Answer from the drawing. Dimensions are ordinates in mm from the lowest x, y and z of the part. Round coordinates to 2 decimals unless told otherwise and drop trailing zeros. Order: outer loops, then holes, each group sorted by start corner. A loop starts at its lowest first (then second) coordinate and runs counter-clockwise, first axis right, second up. Notation, with made-up numbers: (36.25, 36) - (61.25, 36) arc R25 cw to (61.25, 61) - close; hole circle Ø10 at (12.25, 35.5). An arc over 180 degrees is marked (long way). One line per question, with ' | ' between items. Start each with the question number.
1) The part is cut by section C-C, the plane x = 20. Give the vertices of the cut face in (y, z).
2) Flat-ended cylindrical pins translate along their axes: pin 1 (2.5 mm diameter, centred on x = 30, y = 10, fed in from -Z); pin 2 (1.5 mm diameter, centred on y = 47.5, z = 1, fed in from -X). Find the tip coordinate at first contact, or state that the pin passes through.
3) Straight lines are drawn through the part: line 1 (Y direction, x = 20, z = 1.65); line 2 (Y direction, x = 21, z = 2.3); line 3 (X direction, y = 8.5, z = 1.5). For each, find the intervals that lie inside material, in ascending order. Write a range as from..to.
4) The part is cut by section A-A, the plane y = 30. Give the vertices of the cut face in (x, z), plus the area to 3 significant figures.
5) The part is cut by section B-B, the plane y = 10. Give the vertices of the cut face in (x, z).
6) The part is cut by section D-D, the plane z = 2.2. Count the separate pieces of the cut face and the enclosed holes in it, plus the area to 3 significant figures.
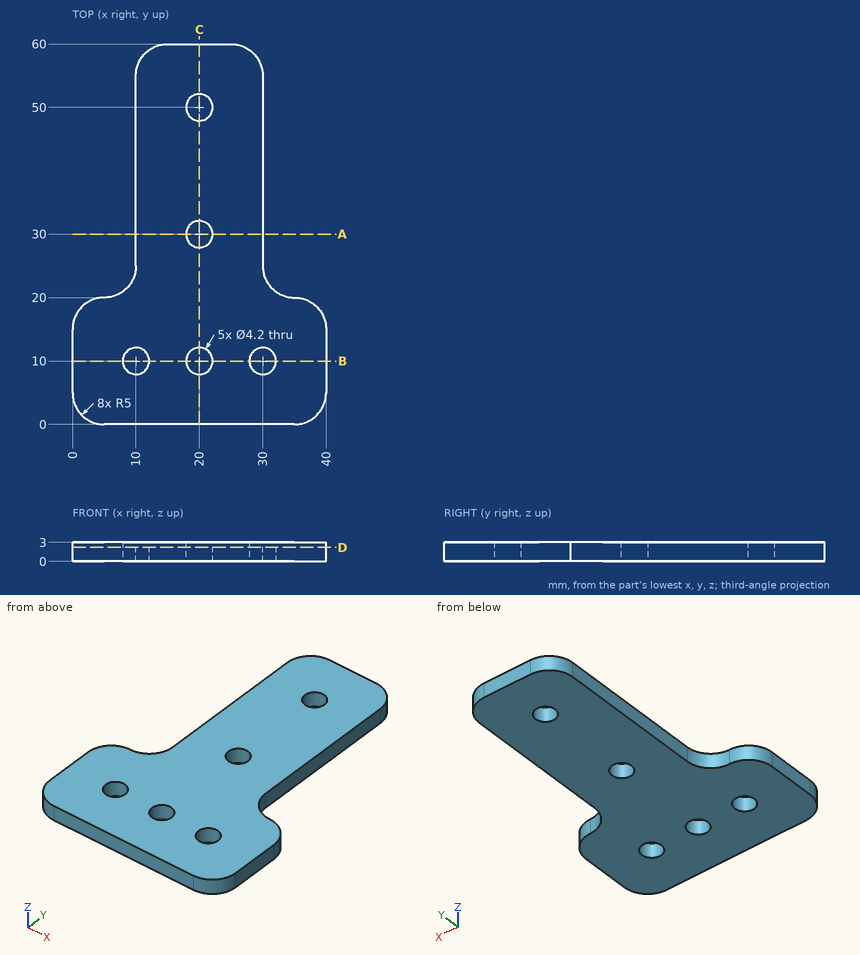
Values:
1) outline: (0, 0) - (7.9, 0) - (7.9, 3) - (0, 3) - close; (12.1, 0) - (27.9, 0) - (27.9, 3) - (12.1, 3) - close; (32.1, 0) - (47.9, 0) - (47.9, 3) - (32.1, 3) - close; (52.1, 0) - (60, 0) - (60, 3) - (52.1, 3) - close
2) pin 1: passes through | pin 2: stops at x = 10
3) line 1: y = 0..7.9, 12.1..27.9, 32.1..47.9, 52.1..60 | line 2: y = 0..8.15, 11.85..28.15, 31.85..48.15, 51.85..60 | line 3: x = 0..8.53, 11.47..18.53, 21.47..28.53, 31.47..40
4) outline: (10, 0) - (17.9, 0) - (17.9, 3) - (10, 3) - close; (22.1, 0) - (30, 0) - (30, 3) - (22.1, 3) - close | area: 47.4 mm^2
5) outline: (0, 0) - (7.9, 0) - (7.9, 3) - (0, 3) - close; (12.1, 0) - (17.9, 0) - (17.9, 3) - (12.1, 3) - close; (22.1, 0) - (27.9, 0) - (27.9, 3) - (22.1, 3) - close; (32.1, 0) - (40, 0) - (40, 3) - (32.1, 3) - close
6) separate pieces: 1 | enclosed holes: 5 | area: 1,510 mm^2
